```python
from build123d import *

# Parameters (mm, degrees)
SKETCH_1_R      = 1.5
SKETCH_1_R_2    = 3
SKETCH_1_R_3    = 1.25
SKETCH_1_R_4    = 2
SKETCH_1_W      = 4.3
SKETCH_1_H      = 8.3
EXTRUDE_1_DEPTH = 4
FILLET_1_R      = 1.3
FILLET_2_R      = 2


with BuildPart() as part:
    # 草图1 → 凸台-拉伸1 (new body)
    with BuildSketch(Plane.XY):
        with BuildLine():
            Line((32.115707856, 27.15), (32.115707856, 22.85))
            Line((32.115707856, 22.85), (27.815707856, 22.85))
            Line((27.815707856, 22.85), (27.815707856, 27.15))
            Line((27.815707856, 27.15), (-29.075, 27.15))
            Line((-29.075, 27.15), (-38.998995168, 22.002009663))
            ThreePointArc((-38.998995168, 22.002009663), (-52.370174504, 17.472835843), (-60.236366221, 5.75))
            Line((-60.236366221, 5.75), (-80.958287312, 5.75))
            Line((-80.958287312, 5.75), (-80.958287312, -5.75))
            Line((-80.958287312, -5.75), (-60.236366221, -5.75))
            ThreePointArc((-60.236366221, -5.75), (-52.370174504, -17.472835843), (-38.998995168, -22.002009663))
            Line((-38.998995168, -22.002009663), (-29.075, -27.15))
            Line((-29.075, -27.15), (27.815707856, -27.15))
            Line((27.815707856, -27.15), (27.815707856, -22.85))
            Line((27.815707856, -22.85), (32.115707856, -22.85))
            Line((32.115707856, -22.85), (32.115707856, -27.15))
            Line((32.115707856, -27.15), (36.001004832, -27.15))
            Line((36.001004832, -27.15), (36.001004832, 27.15))
            Line((36.001004832, 27.15), (32.115707856, 27.15))
        make_face()
        with Locations((30.001004832, 13.5)):
            Circle(SKETCH_1_R, mode=Mode.SUBTRACT)
        with Locations(Location((30.001004832, -13.5, 0), (0, 0, 180))):
            Circle(SKETCH_1_R, mode=Mode.SUBTRACT)
        with Locations((-38.998995168, 0)):
            Circle(SKETCH_1_R_2, mode=Mode.SUBTRACT)
        with Locations((-38.998995168, -11.5)):
            Circle(SKETCH_1_R_3, mode=Mode.SUBTRACT)
        with Locations((-48.958287312, -5.75)):
            Circle(SKETCH_1_R_3, mode=Mode.SUBTRACT)
        with Locations((-48.958287312, 5.75)):
            Circle(SKETCH_1_R_3, mode=Mode.SUBTRACT)
        with Locations((-38.998995168, 11.5)):
            Circle(SKETCH_1_R_3, mode=Mode.SUBTRACT)
        with Locations((-29.039703025, 5.75)):
            Circle(SKETCH_1_R_3, mode=Mode.SUBTRACT)
        with Locations((-29.039703025, -5.75)):
            Circle(SKETCH_1_R_3, mode=Mode.SUBTRACT)
        with Locations((-4.075, -22.15)):
            Circle(SKETCH_1_R_4, mode=Mode.SUBTRACT)
        with Locations((-4.075, 22.15)):
            Circle(SKETCH_1_R_4, mode=Mode.SUBTRACT)
        with Locations((-76.958287312, 0)):
            Circle(SKETCH_1_R_4, mode=Mode.SUBTRACT)
        with Locations((30.001004832, 0)):
            Rectangle(SKETCH_1_W, SKETCH_1_H, mode=Mode.SUBTRACT)
        Polygon((-2.627787708, -13.528909152), (22.001004832, -7.277030256), (22.001004832, 7.277030256), (-2.627787708, 13.528909152), (-21.039703025, 1.433615613), (-21.039703025, -1.433615613), align=None, mode=Mode.SUBTRACT)
    extrude(amount=EXTRUDE_1_DEPTH)

    # 圆角1
    fillet_1_edges = [part.edges().sort_by_distance(p)[0] for p in [
        (-60.236366221, -5.75, 2),
        (-80.958287312, -5.75, 2),
        (-80.958287312, 5.75, 2),
        (-60.236366221, 5.75, 2),
        (36.001004832, 27.15, 2),
        (36.001004832, -27.15, 2),
    ]]
    fillet(fillet_1_edges, radius=FILLET_1_R)

    # 圆角2
    fillet_2_edges = [part.edges().sort_by_distance(p)[0] for p in [
        (-21.039703025, -1.433615613, 2),
        (-2.627787708, -13.528909152, 2),
        (22.001004832, -7.277030256, 2),
        (22.001004832, 7.277030256, 2),
        (-2.627787708, 13.528909152, 2),
        (-21.039703025, 1.433615613, 2),
    ]]
    fillet(fillet_2_edges, radius=FILLET_2_R)


solid = part.part
```
Check sheet for the modelled part. Datum: model origin and axes. Units: mm. A direction names the side the tool comes from. Give positions to 0.01 mm unless a question says otherwise; leave off trailing zeros. Loops run counter-clockwise (first coordinate to the right, second up) from the corner with the lowest first, then second, coordinate; pieces in that order, holes last. Notation, with made-up numbers: M 82.5,36 L 98.5,36 A34 ccw 98.5,75 Z; hole C 75,52.25 d7. An arc over 180 degrees is marked long. Answer in a Markdown table with one row per item.
1) Mould release check, pull along X, two halves, no side actions. Record for faces 6 (the face through (-38.327, 12.554, 1.972)), 7 (the face through (-1, -27.15, 2)), 8 (the face through (-52.15, -17.64, 1.97)): released by +X, released by -X, zero draft, split by the parting line, or undercut.
Solutions:
| item | result |
|---|---|
| face 6 | undercut |
| face 7 | zero draft |
| face 8 | released by -X |
2) Thickness scan on line 1 (Y direction, x = -49.5, z = 3.8); line 2 (Y direction, x = 29, z = 1.4); line 3 (Y direction, x = -5, z = 1.55). Record the ranges inside material, lowest first.
Solutions:
| item | result |
|---|---|
| line 1 | y = -19.33 to -6.88, -4.62 to 4.62, 6.88 to 19.33 |
| line 2 | y = -22.85 to -14.62, -12.38 to -4.15, 4.15 to 12.38, 14.62 to 22.85 |
| line 3 | y = -27.15 to -23.92, -20.38 to -11.97, 11.97 to 20.38, 23.92 to 27.15 |
3) Depth check by flat-ended pin: pin 1 (2 mm diameter, centred on x = 20.5, y = -13.5, fed in from -Z); pin 2 (2 mm diameter, centred on x = 29, z = 2, fed in from -Y). Enter the tip coordinate at first touch or a pass-through.
Solutions:
| item | result |
|---|---|
| pin 1 | stops at z = 0 |
| pin 2 | stops at y = -22.85 |
4) Cross-section at A-A (x = 6). Enter the section's corners in (y, z).
Solutions:
| item | result |
|---|---|
| outline | M -27.15,0 L -11.34,0 L -11.34,4 L -27.15,4 Z; M 11.34,0 L 27.15,0 L 27.15,4 L 11.34,4 Z |
5) Cross-section at C-C (x = -66). Enter the section's corners in (y, z), plus the area to 3 significant figures.
Solutions:
| item | result |
|---|---|
| outline | M -5.75,0 L 5.75,0 L 5.75,4 L -5.75,4 Z |
| area | 46.0 mm^2 |
6) Cross-section at D-D (x = -45). Enter the section's corners in (y, z).
Solutions:
| item | result |
|---|---|
| outline | M -21.17,0 L 21.17,0 L 21.17,4 L -21.17,4 Z |
7) Cross-section at B-B (z = 1.2). Count the separate pieces of the cut face and the enclosed holes in it, plus the area to 3 significant figures.
Solutions:
| item | result |
|---|---|
| separate pieces | 1 |
| enclosed holes | 14 |
| area | 4,040 mm^2 |
8) Tool access check on faces 1 (the face through (32.116, -25, 2)), 2 (the face through (-70, 5.75, 2)), 3 (the face through (-71, -5.75, 2)), 4 (the face through (27.816, 25, 2)), 5 (the face through (9.515, 10.446, 1.972)). Record the directions out of +Z, -Z, +X, -X, +Y, -Y that give a thin tool (end or side, any length) a straight path to the whole face; none if there is none.
Solutions:
| item | result |
|---|---|
| face 1 | +Z, -Z, -Y |
| face 2 | +Z, -Z, -X, +Y |
| face 3 | +Z, -Z, -X, -Y |
| face 4 | +Z, -Z, +Y |
| face 5 | +Z, -Z |
